Source: three-view drawing plus pictorial views. Frame: mm from the lowest corner of the part. A direction names the side the tool comes from. Round coordinates to 2 decimals unless told otherwise and drop trailing zeros. Loops run counter-clockwise (first coordinate to the right, second up) from the corner with the lowest first, then second, coordinate; pieces in that order, holes last. Notation, with made-up numbers: M 42.25,17.25 L 62.25,17.25 A21 cw 62.25,36.25 Z; hole C -16,-5.5 d8. An arc over 180 degrees is marked long. Return JSON: item names as keys, results as strings. Group by question number.
1) Section D-D (x = 52.5). Output: boundary loops of the cut face in (y, z).
2) Section B-B (x = 116.5). Output: boundary loops of the cut face in (y, z).
3) Contact query for flat-ended pins moving along their axis: P1, Ø6, axis at x = 70, z = 116.5, coming from the +Y side; P2, Ø8, axis at y = 51, z = 22, coming from the +X side; P3, Ø1, axis at x = 93.5, z = 87.5, coming from the +Y side. Output: stop coordinate, or through.
4) Material intervals for line 1 (Y direction, x = 69, z = 56); line 2 (X direction, y = 171.5, z = 110); line 3 (Y direction, x = 107, z = 45), sorted ascending. Write a range as from..to.
5) Section C-C (y = 106). Output: boundary loops of the cut face in (x, z).
6) Mould query, pull axis Z, two halves, no side actions, for the marked faces 1, 2, 3 and 4. Classes: +Z half, -Z half, draft (parallel to the pull), parting line (faces both ways), or undercut.
7) Access query for the marked faces 5, 6 and 7. Directions: +Z, -Z, +X, -X, +Y, -Y. A direction counts if a zero-diameter tool reaches every point of the face in a straight line with its end or side. Return the directions, or none.
8) Section A-A (z = 13). Output: boundary loops of the cut face in (x, y).
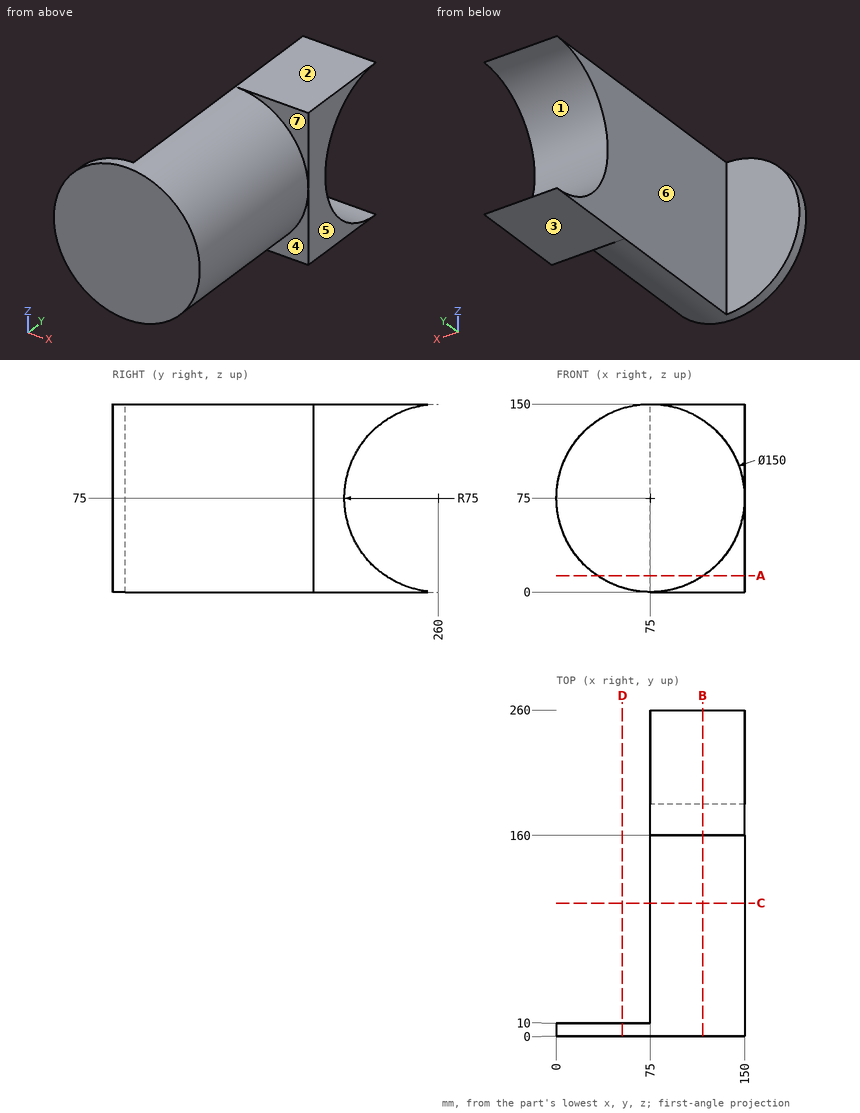
Returned:
{
 "1": {"outline": "M 0,3.45 L 10,3.45 L 10,146.55 L 0,146.55 Z"},
 "2": {"outline": "M 0,12.53 L 160,12.53 L 160,0 L 260,0 A75 cw 260,150 L 160,150 L 160,137.47 L 0,137.47 Z"},
 "3": {"P1": "stops at y = 10", "P2": "stops at x = 131.78", "P3": "stops at y = 186.14"},
 "4": {"line 1": "y = 0..10", "line 2": "x = 75..150", "line 3": "y = 0..191.26"},
 "5": {"outline": "M 75,0 A75 ccw 75,150 Z"},
 "6": {"face 1": "undercut", "face 2": "+Z half", "face 3": "-Z half", "face 4": "draft"},
 "7": {"face 5": "+Z, -Z, +X, +Y, -Y", "face 6": "+Z, -Z, -X, +Y", "face 7": "+Z, +X, -Y"},
 "8": {"outline": "M 32.8,0 L 117.2,0 L 117.2,160 L 150,160 L 150,217.8 L 75,217.8 L 75,10 L 32.8,10 Z"}
}
